Work out the finished part from the listing and answer in its coordinate system (mm). Face numbers are marked on the shaded views. Coordinates: 2 decimals unless noted, no trailing zeros. Order: outer loops, then holes, each group sorted by start corner. A loop starts at its lowest first (then second) coordinate and runs counter-clockwise, first axis right, second up. Notation, with made-up numbers: (23.5, -11.5) - (43.5, -11.5) arc R12 ccw to (43.5, 0.5) - close; hole circle Ø3 at (39, 6.5). An arc over 180 degrees is marked (long way). Answer as a JSON object with one key per item and string values. Group by question number.
1) Section A-A (z = 13.5) is taken. Give the vertices of the cut face in (x, y).
2) Each of these flat-tipped pins is pushed along its axis until it touches: P1, Ø10, axis at x = -1.5, z = -9, coming from the -Y side; P2, Ø2, axis at y = -1.5, z = 11, coming from the -X side; P3, Ø2, axis at x = 9.5, z = -6.5, coming from the +Y side. Where does it stop, or does it pass through?
3) The mould has two halves that part along Z. Classify the marked faces 1, 2 and 3: released by +Z, released by -Z, zero draft, split by the parting line, or undercut.
4) Find the intervals of material crossed by line 1 along Y through (x, z) = (11.25, 5); line 2 along X through (y, z) = (0, 14.5); line 3 along X through (y, z) = (9.75, 6.5), in increasing order.
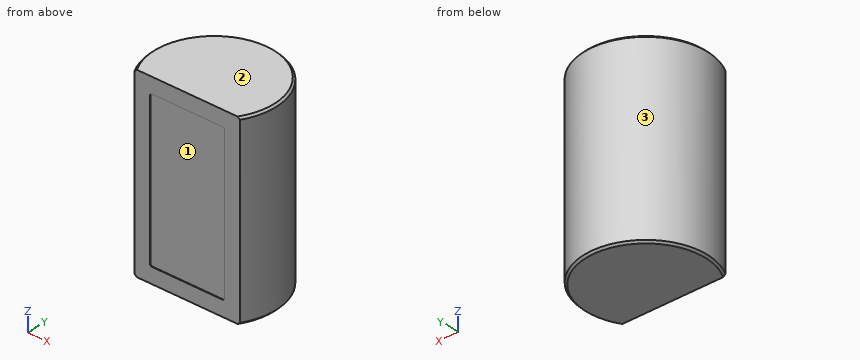
from build123d import *

# Parameters (mm, degrees)
SKETCH1_R            = 12.7
EXTRUDE1_DEPTH       = 19.05
CHAMFER1_SIZE        = 0.4064
TRUNCATED_DEPTH      = 20.05
TRUNCATED_DEPTH_BACK = 20.05
RECESSED_DEPTH       = 0.127


with BuildPart() as part:
    # Sketch1 → Extrude1 (new body, symmetric)
    with BuildSketch(Plane.XY):
        Circle(SKETCH1_R)
    extrude(amount=EXTRUDE1_DEPTH, both=True)

    # Chamfer1
    chamfer1_edges = [part.edges().sort_by_distance(p)[0] for p in [
        (-12.7, 0, -19.05),
        (-12.7, 0, 19.05),
    ]]
    chamfer(chamfer1_edges, length=CHAMFER1_SIZE)

    # Sketch2 → Truncated (cut, two sides)
    with BuildSketch(Plane.XY) as truncated_sk:
        with BuildLine():
            Line((-10.998522628, -6.35), (10.998522628, -6.35))
            ThreePointArc((10.998522628, -6.35), (0, -12.7), (-10.998522628, -6.35))
        make_face()
    extrude(amount=TRUNCATED_DEPTH, mode=Mode.SUBTRACT)
    extrude(truncated_sk.sketch, amount=-TRUNCATED_DEPTH_BACK, mode=Mode.SUBTRACT)

    # Sketch3 → Recessed (cut)
    with BuildSketch(Plane.XZ.offset(6.35)):
        with BuildLine():
            Line((7.315522628, 15.875), (-7.315522628, 15.875))
            ThreePointArc((-7.315522628, 15.875), (-7.674732873, 15.726210245), (-7.823522628, 15.367))
            Line((-7.823522628, 15.367), (-7.823522628, -15.367))
            ThreePointArc((-7.823522628, -15.367), (-7.674732873, -15.726210245), (-7.315522628, -15.875))
            Line((-7.315522628, -15.875), (7.315522628, -15.875))
            ThreePointArc((7.315522628, -15.875), (7.674732873, -15.726210245), (7.823522628, -15.367))
            Line((7.823522628, -15.367), (7.823522628, 15.367))
            ThreePointArc((7.823522628, 15.367), (7.674732873, 15.726210245), (7.315522628, 15.875))
        make_face()
    extrude(amount=-RECESSED_DEPTH, mode=Mode.SUBTRACT)


solid = part.part
Report:
{
 "1": {"outline": "(-11, -6.35) - (-7.82, -6.35) - (-7.82, -6.22) - (7.82, -6.22) - (7.82, -6.35) - (11, -6.35) arc R12.7 ccw (long way) to start"},
 "2": {"P1": "stops at y = -6.22", "P2": "stops at x = -12.69", "P3": "stops at y = 9.44"},
 "3": {"face 1": "undercut", "face 2": "released by +Z", "face 3": "zero draft"},
 "4": {"line 1": "y = -5.89 to 5.89", "line 2": "x = -12.7 to 12.7", "line 3": "x = -8.14 to 8.14"}
}
